The model under review builds one solid part; all positions refer to its coordinate system, in mm. A direction names the side the tool comes from. Round coordinates to 2 decimals unless told otherwise and drop trailing zeros. Answer as a JSON object with one key per item and string values. Group by question number.
1) Insertion check: pin 1 Ø10 at (x, z) = (-8, 31.5) entering from -Y; pin 2 Ø6 at (x, z) = (8, 36) entering from +Y; pin 3 Ø3 at (x, z) = (3, 15) entering from -Y. Each pin has a flat end and moves straight along its axis. Give the tip position at first contact, or say it passes through.
2) Machinability: for faces 1 (the flat face through (1, 0, 44)), 2 (the flat face through (0, 0, 29)), which of the approach directions +Z, -Z, +X, -X, +Y, -Y give a long, thin tool a straight path to every point of the face, cutting with its end or side? Answer none if there is none.
3) To check wall thickness, follow probe 1 along X at (y, z) = (-1.75, 35); probe 2 along X at (y, z) = (-0.25, 39); probe 3 along Z at (x, y) = (-9.25, 1.25). State the ranges of each line that lie inside material, in increasing order. Write a range as [from, to].
4) Mouldability with a two-part tool opening along Y and no side actions: class faces 3 (the flat face through (0, 0, 0)), 4 (the cylindrical face through (-0.867, -3.905, 40.958)), 5 (the flat face through (0.7, 0, 37)) as pulls with the +Y half, pulls with the -Y half, needs draft (parallel to the pull), parting line crosses it, or undercut.
from build123d import *

# Parameters (mm, degrees)
F4_R     = 4
F5_DEPTH = 6
F7_DEPTH = 15


with BuildPart() as f3:
    # F0 (on Top) → F3 section 0
    with BuildSketch(Plane.XY):
        Polygon((12.5, 1.5), (0, 2.25), (-12.5, 1.5), (-12.5, 0), (-12.5, -1.5), (0, -2.25), (12.5, -1.5), (12.5, 0), align=None)
    # F2 (on offset) → F3 section 1
    with BuildSketch(Plane.XY.offset(38)):
        Polygon((-12.5, 3.25), (-12.5, 0), (-12.5, -3.25), (0, -5), (12.5, -3.25), (12.5, 0), (12.5, 3.25), (0, 5), align=None)
    loft()

    # F4 (on face) → F5 (join)
    with BuildSketch(Plane.XY.offset(38)):
        Circle(F4_R)
    extrude(amount=F5_DEPTH)

    # F6 (on face) → F7 (cut)
    with BuildSketch(Plane.XY.offset(44)):
        with BuildLine():
            Line((-0.7, 2.3), (-0.7, 0))
            Line((-0.7, 0), (-0.7, -2.3))
            ThreePointArc((-0.7, -2.3), (-0.4949747468, -2.7949747468), (0, -3))
            ThreePointArc((0, -3), (0.4949747468, -2.7949747468), (0.7, -2.3))
            Line((0.7, -2.3), (0.7, 0))
            Line((0.7, 0), (0.7, 2.3))
            ThreePointArc((0.7, 2.3), (0.4949747468, 2.7949747468), (0, 3))
            ThreePointArc((0, 3), (-0.4949747468, 2.7949747468), (-0.7, 2.3))
        make_face()
    extrude(amount=-F7_DEPTH, mode=Mode.SUBTRACT)


solid = f3.part
Here are the results:
{
 "1": {"pin 1": "stops at y = -4.23", "pin 2": "stops at y = 4.22", "pin 3": "stops at y = -3.23"},
 "2": {"face 1": "+Z, +X, -X, +Y, -Y", "face 2": "+Z"},
 "3": {"probe 1": "x = [-12.5, -0.7], [0.7, 12.5]", "probe 2": "x = [-3.99, -0.7], [0.7, 3.99]", "probe 3": "z = [0, 38]"},
 "4": {"face 3": "needs draft", "face 4": "parting line crosses it", "face 5": "undercut"}
}
